from build123d import *

# Parameters (mm, degrees)
SKETCH_W     = 28.4
SKETCH_H     = 11.6
SKETCH_R     = 1
SKETCH_W_2   = 19.3
SKETCH_H_2   = 8
PAD_DEPTH    = 4
SKETCH001_R  = 1.6
PAD001_DEPTH = 2


with BuildPart() as part:
    # Sketch → Pad (new body)
    with BuildSketch(Plane.XY):
        Rectangle(SKETCH_W, SKETCH_H)
        with Locations((-11.7, 3.3)):
            Circle(SKETCH_R, mode=Mode.SUBTRACT)
        with Locations((11.7, -3.3)):
            Circle(SKETCH_R, mode=Mode.SUBTRACT)
        Rectangle(SKETCH_W_2, SKETCH_H_2, mode=Mode.SUBTRACT)
    extrude(amount=PAD_DEPTH)

    # Sketch001 → Pad001 (new body)
    with BuildSketch(Plane.XY.offset(4)):
        with BuildLine():
            Line((-14.2, 2.8), (-32, 2.8))
            ThreePointArc((-32, 8.8), (-35, 5.8), (-32, 2.8))
            Line((-32, 8.8), (32, 8.8))
            ThreePointArc((32, 2.8), (35, 5.8), (32, 8.8))
            Line((32, 2.8), (14.2, 2.8))
            Line((14.2, 2.8), (14.2, 5.7))
            Line((14.2, 5.7), (-14.2, 5.7))
            Line((-14.2, 5.7), (-14.2, 2.8))
        make_face()
        with Locations((-32, 5.8)):
            Circle(SKETCH001_R, mode=Mode.SUBTRACT)
        with Locations((32, 5.8)):
            Circle(SKETCH001_R, mode=Mode.SUBTRACT)
    extrude(amount=-PAD001_DEPTH)


solid = part.part
Source: CAD feature listing. Evaluate the final solid. Frame: model axes, mm. A direction names the side the tool comes from. Round coordinates to 2 decimals unless told otherwise and drop trailing zeros. Loops run counter-clockwise (first coordinate to the right, second up) from the corner with the lowest first, then second, coordinate; pieces in that order, holes last.
Q1. First-contact query: P1, Ø2, axis at x = -21, z = 3, coming from the -Y side; P2, Ø2, axis at y = 3.5, z = 3, coming from the -X side; P3, Ø2, axis at y = 0.5, z = 1.5, coming from the +X side. Flat tips, straight axial feed; report the tip coordinate or a pass-through.
Q2. Section B-B, the plane y = -3.3. Return loops of the section in (x, z).
Q3. Section A-A, the plane z = 2.65. Return loops of the section in (x, y).
Q4. Section C-C, the plane x = 11.7. Return loops of the section in (y, z), plus the area to 3 significant figures.
Q5. Section D-D, the plane x = -23. Return loops of the section in (y, z).
Q6. Access query for faces 1 (the face through (-23, 2.8, 3)), 2 (the face through (23, 2.8, 3)), 3 (the face through (14.2, 0, 2)), 4 (the face through (0, 4, 2)), 5 (the face through (-14.2, 0, 2)). Directions: +Z, -Z, +X, -X, +Y, -Y. A direction counts if a zero-diameter tool reaches every point of the face in a straight line with its end or side. Return the directions, or none.
Q7. Mould query, pull axis Y, two halves, no side actions, for faces 6 (the face through (-3, 5, 0)), 7 (the face through (0, 5.8, 1)), 8 (the face through (30.73, 4.83, 3.01)). Classes: pulls with the +Y half, pulls with the -Y half, needs draft (parallel to the pull), parting line crosses it, or undercut.
Q8. Ray query, line 1 (Y direction, x = 11.7, z = 3.2); line 2 (Y direction, x = -11.7, z = 2.2); line 3 (X direction, y = 1, z = 0.65). Return the intervals inside material, ascending.
Solutions:
1. P1: stops at y = 2.8
1. P2: stops at x = -34.7
1. P3: stops at x = 14.2
2. outline: (-14.2, 0) - (-9.65, 0) - (-9.65, 4) - (-14.2, 4) - close; (9.65, 0) - (10.7, 0) - (10.7, 4) - (9.65, 4) - close; (12.7, 0) - (14.2, 0) - (14.2, 4) - (12.7, 4) - close
3. outline: (-32, 2.8) - (-14.2, 2.8) - (-14.2, -5.8) - (14.2, -5.8) - (14.2, 2.8) - (32, 2.8) arc R3 ccw to (32, 8.8) - (-32, 8.8) arc R3 ccw to start; hole circle Ø3.2 at (-32, 5.8); hole circle Ø2 at (-11.7, 3.3); hole (-9.65, -4) - (9.65, -4) - (9.65, 4) - (-9.65, 4) - close; hole circle Ø2 at (11.7, -3.3); hole circle Ø3.2 at (32, 5.8)
4. outline: (-5.8, 0) - (-4.3, 0) - (-4.3, 4) - (-5.8, 4) - close; (-2.3, 0) - (5.8, 0) - (5.8, 2) - (8.8, 2) - (8.8, 4) - (-2.3, 4) - close
4. area: 44.4 mm2
5. outline: (2.8, 2) - (8.8, 2) - (8.8, 4) - (2.8, 4) - close
6. face 1: +Z, -Z, -X, -Y
6. face 2: +Z, -Z, +X, -Y
6. face 3: -Z, +X, -Y
6. face 4: +Z, -Z
6. face 5: -Z, -X, -Y
7. face 6: needs draft
7. face 7: pulls with the +Y half
7. face 8: undercut
8. line 1: y = -5.8 to -4.3, -2.3 to 8.8
8. line 2: y = -5.8 to 2.3, 4.3 to 8.8
8. line 3: x = -14.2 to -9.65, 9.65 to 14.2
